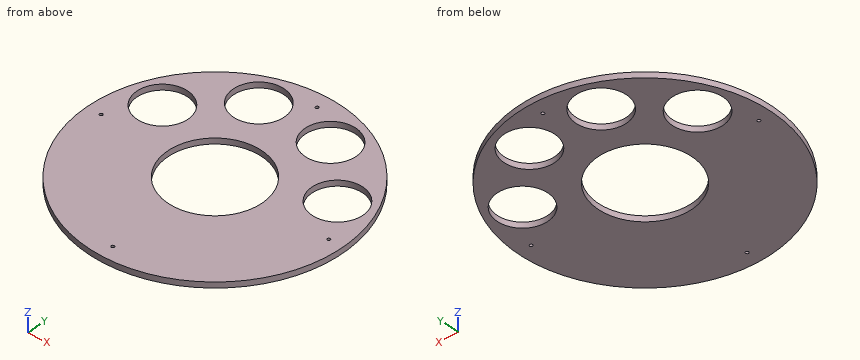
Autodesk Inventor part; units mm, degrees
ref_plane "YZ Plane" through (0, 0, 0) normal (1, 0, 0) x (0, 1, 0)
ref_plane "XZ Plane" through (0, 0, 0) normal (0, 1, 0) x (-1, 0, 0)
ref_plane "XY Plane" through (0, 0, 0) normal (0, 0, 1) x (1, 0, 0)
ref_plane "РабПлоскость1" through (0, 120, 53) normal (0, 0, 1) x (-1, 0, 0)
sketch "Эскиз1" plane through (0, 120, 53) normal (0, 0, 1) x (-1, 0, 0)
  circle A0 centre (0, 120) radius 135
  circle A1 centre (0, 0) radius 1.6
  circle A2 centre (-120, 120) radius 1.6
  circle A3 centre (120, 120) radius 1.6
  circle A4 centre (0, 240) radius 1.6
  circle A5 centre (0, 120) radius 135
  circle A6 centre (37.8353, 26.3544) radius 27
  circle A7 centre (92.2681, 78.9196) radius 27
  circle A8 centre (-37.8353, 26.3544) radius 27
  circle A9 centre (-92.2681, 78.9196) radius 27
  circle A10 centre (0, 120) radius 50
  circle A11 centre (48.4361, 96.1266) radius 1.7
  circle A12 centre (3.5431, 66.1164) radius 1.7
  circle A13 centre (-44.8931, 89.9898) radius 1.7
  circle A14 centre (-48.4361, 143.8734) radius 1.7
  circle A15 centre (-3.5431, 173.8836) radius 1.7
  circle A16 centre (44.8931, 150.0102) radius 1.7
extrude "Выдавливание1" add sketch "Эскиз1" along normal blind 6 contours A0 | A10 | A11 | A12 | A13 | A14 | A15 | A16
sketch "Эскиз2" plane through (0, 0, 59) normal (0, 0, 1) x (1, 0, 0)
  circle A0 centre (0, 0) radius 50
extrude "Выдавливание2" cut sketch "Эскиз2" against normal through all
properties part number "Диск_фиксирующий" material "По умолчанию1"
Here's how the part is built. I have some questions about the finished solid (model axes, mm). Give positions to 0.01 mm unless a question says otherwise; leave off trailing zeros. Loops run counter-clockwise (first coordinate to the right, second up) from the corner with the lowest first, then second, coordinate; pieces in that order, holes last. Notation, with made-up numbers: (-25.5, 7.5) -> (-19.5, 7.5) arc R33 cw to (-19.5, 43.5) -> close; hole circle Ø10 at (-4, 18). An arc over 180 degrees is marked (long way). Use one line per item in the form item = value. Start each with the question number.
1) Imagine slicing it at A-A (x = 82). Please give me the cut outline in (y, z).
2) Imagine slicing it at B-B (y = 111). Please give me the cut outline in (x, z), then the cut area to 3 significant figures.
3) For P1, Ø3, axis at x = 87.5, z = 56, coming from the -Y side; P2, Ø2, axis at x = -22.5, z = 55.5, coming from the -Y side; P3, Ø1, axis at x = -42.5, z = 57, coming from the -Y side, each with a flat end and sliding along its axis, tell me the tip position at first contact or that it passes through.
4) Imagine slicing it at D-D (x = -41). Please give me the cut outline in (y, z), then the cut area to 3 significant figures.
5) Imagine slicing it at C-C (z = 54.65). Count the separate pieces of the cut face and the enclosed holes in it, then the cut area to 3 significant figures.
6) Please list where these lines run through material, in increasing order: line 1 along X through (y, z) = (86.5, 55.65); line 2 along Y through (x, z) = (-28, 57.5); line 3 along X through (y, z) = (91.5, 55.1).
Check values:
q1.outline = (-107.24, 53) -> (16.11, 53) -> (16.11, 59) -> (-107.24, 59) -> close; (66.05, 53) -> (107.24, 53) -> (107.24, 59) -> (66.05, 59) -> close
q2.outline = (-76.84, 53) -> (-58.52, 53) -> (-58.52, 59) -> (-76.84, 59) -> close; (-17.15, 53) -> (17.15, 53) -> (17.15, 59) -> (-17.15, 59) -> close; (58.52, 53) -> (76.84, 53) -> (76.84, 59) -> (58.52, 59) -> close
q2.area = 426 mm^2
q3.P1 = -104.06
q3.P2 = -133.28
q3.P3 = -128.3
q4.outline = (-128.62, 53) -> (-28.62, 53) -> (-28.62, 59) -> (-128.62, 59) -> close; (28.62, 53) -> (66.83, 53) -> (66.83, 59) -> (28.62, 59) -> close; (120.46, 53) -> (128.62, 53) -> (128.62, 59) -> (120.46, 59) -> close
q4.area = 878 mm^2
q5.separate_pieces = 1
q5.enclosed_holes = 9
q5.area = 40,200 mm^2
q6.line_1 = -103.65 to -63.87, -11.8 to 11.8, 63.87 to 103.65
q6.line_2 = -132.06 to -41.42, 41.42 to 68.5, 118.79 to 132.06
q6.line_3 = -99.26 to -64.75, -10.92 to 10.92, 64.75 to 99.26
